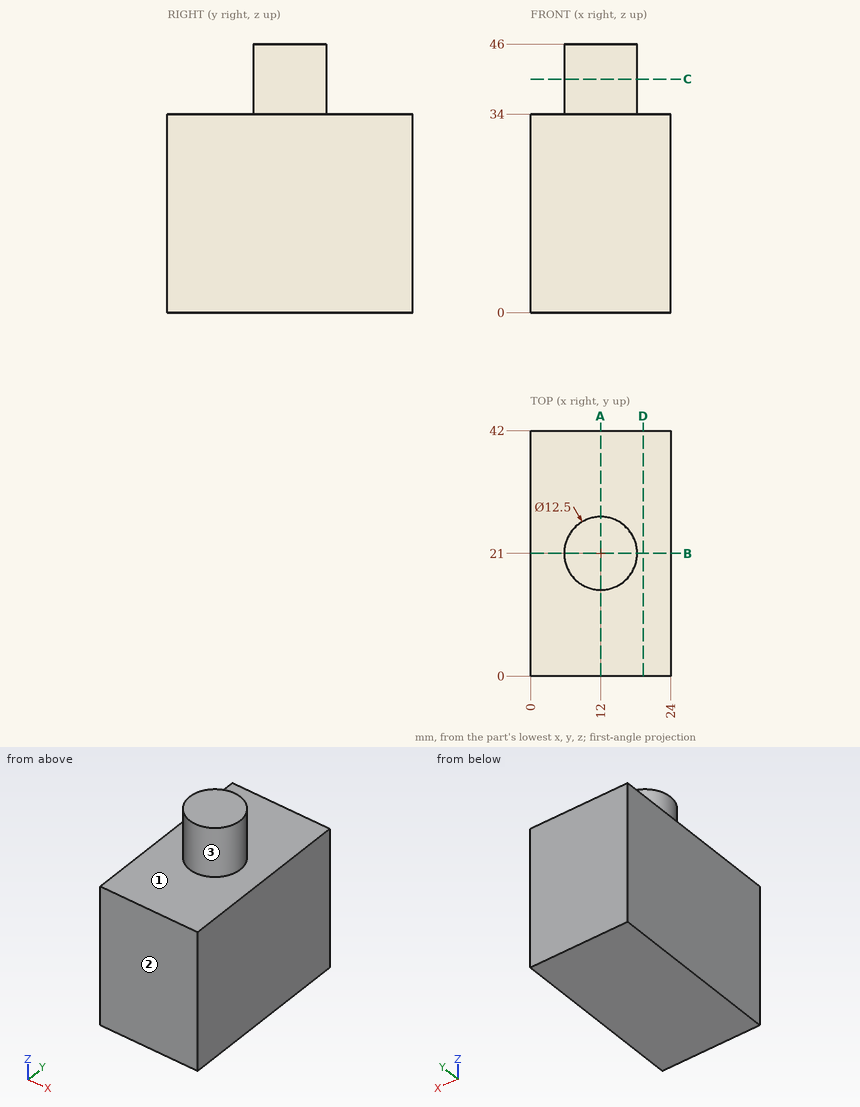
Source: three-view drawing plus pictorial views. Frame: mm from the lowest corner of the part. Give positions to 0.01 mm unless a question says otherwise; leave off trailing zeros. Loops run counter-clockwise (first coordinate to the right, second up) from the corner with the lowest first, then second, coordinate; pieces in that order, holes last.
1) Section query B-B on y = 21. Return the cut outline in (x, z).
A:
outline: (0, 0) - (24, 0) - (24, 34) - (18.25, 34) - (18.25, 46) - (5.75, 46) - (5.75, 34) - (0, 34) - close
2) Section query A-A on x = 12. Return the cut outline in (y, z).
A:
outline: (0, 0) - (42, 0) - (42, 34) - (27.25, 34) - (27.25, 46) - (14.75, 46) - (14.75, 34) - (0, 34) - close
3) Section query C-C on z = 40. Return the cut outline in (x, y).
A:
outline: circle Ø12.5 at (12, 21)
4) Contact query for flat-ended pins moving along their axis: pin 1 (1 mm diameter, centred on x = 7.5, y = 12, fed in from +Z); pin 2 (5 mm diameter, centred on y = 21, z = 41, fed in from +X); pin 3 (6 mm diameter, centred on x = 11.5, z = 39, fed in from +Y). Output: stop coordinate, or through.
A:
pin 1: stops at z = 34
pin 2: stops at x = 18.25
pin 3: stops at y = 27.25
5) Line query: L1, parallel to Z at x = 3.25, y = 17.5; L2, parallel to X at y = 26, z = 40; L3, parallel to X at y = 21.5, z = 38.5. Output: solid intervals per line, ascending.
A:
L1: z = 0 to 34
L2: x = 8.25 to 15.75
L3: x = 5.77 to 18.23
6) Section query D-D on x = 19.25. Return the cut outline in (y, z), and give its area (3 significant figures).
A:
outline: (0, 0) - (42, 0) - (42, 34) - (0, 34) - close
area: 1,430 mm2
7) Mould query, pull axis Y, two halves, no side actions, for the marked faces 1, 2 and 3. Classes: released by +Y, released by -Y, zero draft, split by the parting line, or undercut.
A:
face 1: zero draft
face 2: released by -Y
face 3: split by the parting line
